Can you work these out from the model? Positions are in its coordinate system, mm. Face numbers are marked on the shaded views. A direction names the side the tool comes from. Give positions to 0.01 mm unless a question says otherwise; leave off trailing zeros. Order: outer loops, then holes, each group sorted by start corner. A loop starts at its lowest first (then second) coordinate and runs counter-clockwise, first axis right, second up.
Item 1: I want a section at A-A, the plane y = 141. Write out the boundary of the cut face in (x, z).
Item 2: If we mould it in two halves opening along X, with no side actions, what happens to the marked faces 4, 5 and 6? For each: +X half, -X half, draft (parallel to the pull), parting line (faces both ways), or undercut.
Item 3: Which directions (+Z, -Z, +X, -X, +Y, -Y) give clear straight access to the entire face, cutting with the end or side of a thin tool? Please do the marked faces 1, 2 and 3.
Item 4: If I drill on line 1 along X through (y, z) = (8, 0) (3 decimals); line 2 along Z through (x, y) = (63, 3); line 3 along Y through (x, z) = (-117, 68), over which ranges is the centre line in solid material (lowest first)?
Item 5: I'm going to push flat-ended pins straight in: pin 1 Ø10 at (y, z) = (93.5, -39.5) entering from +X; pin 2 Ø8 at (y, z) = (82.5, 90.5) entering from -X; pin 3 Ø5 at (x, z) = (109.99, 63.5) entering from +Y; pin 4 Ø6 at (y, z) = (215.5, -49) entering from +X. Where does each tip first touch, or does it pass through?
Item 6: I want a section at B-B, the plane y = 52. Write out the boundary of the cut face in (x, z), then the cut area to 3 significant figures.
```python
from build123d import *

# Parameters (mm, degrees)
SKETCH2_R           = 101.6
SKETCH2_R_2         = 69.85
SKETCH2_R_3         = 3.175
BOSS_EXTRUDE1_DEPTH = 12.7
SKETCH3_R           = 139.7
SKETCH3_R_2         = 107.95
SKETCH3_R_3         = 3.175
BOSS_EXTRUDE2_DEPTH = 12.7


with BuildPart() as part:
    # Sketch1 → Revolve1 (revolve)
    with BuildSketch(Plane.XY):
        Polygon((69.85, 279.4), (107.95, 0), (114.3, 0), (76.2, 279.4), align=None)
    revolve(axis=Axis((0, 279.4, 0), (0, -1, 0)))

    # Sketch2 → Boss-Extrude1 (add)
    with BuildSketch(Plane(origin=(0, 279.4, 0), x_dir=(1, 0, 0), z_dir=(0, 1, 0))):
        Circle(SKETCH2_R)
        Circle(SKETCH2_R_2, mode=Mode.SUBTRACT)
        with Locations((0, 88.9)):
            Circle(SKETCH2_R_3, mode=Mode.SUBTRACT)
        with Locations((44.45, 76.989658396)):
            Circle(SKETCH2_R_3, mode=Mode.SUBTRACT)
        with Locations((76.989658396, 44.45)):
            Circle(SKETCH2_R_3, mode=Mode.SUBTRACT)
        with Locations((88.9, 0)):
            Circle(SKETCH2_R_3, mode=Mode.SUBTRACT)
        with Locations((76.989658396, -44.45)):
            Circle(SKETCH2_R_3, mode=Mode.SUBTRACT)
        with Locations((44.45, -76.989658396)):
            Circle(SKETCH2_R_3, mode=Mode.SUBTRACT)
        with Locations((0, -88.9)):
            Circle(SKETCH2_R_3, mode=Mode.SUBTRACT)
        with Locations((-44.45, -76.989658396)):
            Circle(SKETCH2_R_3, mode=Mode.SUBTRACT)
        with Locations((-76.989658396, -44.45)):
            Circle(SKETCH2_R_3, mode=Mode.SUBTRACT)
        with Locations((-88.9, 0)):
            Circle(SKETCH2_R_3, mode=Mode.SUBTRACT)
        with Locations((-76.989658396, 44.45)):
            Circle(SKETCH2_R_3, mode=Mode.SUBTRACT)
        with Locations((-44.45, 76.989658396)):
            Circle(SKETCH2_R_3, mode=Mode.SUBTRACT)
    extrude(amount=-BOSS_EXTRUDE1_DEPTH)

    # Sketch3 → Boss-Extrude2 (add)
    with BuildSketch(Plane(origin=(0, 0, 0), x_dir=(-1, 0, 0), z_dir=(0, -1, 0))):
        Circle(SKETCH3_R)
        Circle(SKETCH3_R_2, mode=Mode.SUBTRACT)
        with Locations((0, 127)):
            Circle(SKETCH3_R_3, mode=Mode.SUBTRACT)
        with Locations((63.5, 109.985226281)):
            Circle(SKETCH3_R_3, mode=Mode.SUBTRACT)
        with Locations((109.985226281, 63.5)):
            Circle(SKETCH3_R_3, mode=Mode.SUBTRACT)
        with Locations((127, 0)):
            Circle(SKETCH3_R_3, mode=Mode.SUBTRACT)
        with Locations((109.985226281, -63.5)):
            Circle(SKETCH3_R_3, mode=Mode.SUBTRACT)
        with Locations((63.5, -109.985226281)):
            Circle(SKETCH3_R_3, mode=Mode.SUBTRACT)
        with Locations((0, -127)):
            Circle(SKETCH3_R_3, mode=Mode.SUBTRACT)
        with Locations((-63.5, -109.985226281)):
            Circle(SKETCH3_R_3, mode=Mode.SUBTRACT)
        with Locations((-109.985226281, -63.5)):
            Circle(SKETCH3_R_3, mode=Mode.SUBTRACT)
        with Locations((-127, 0)):
            Circle(SKETCH3_R_3, mode=Mode.SUBTRACT)
        with Locations((-109.985226281, 63.5)):
            Circle(SKETCH3_R_3, mode=Mode.SUBTRACT)
        with Locations((-63.5, 109.985226281)):
            Circle(SKETCH3_R_3, mode=Mode.SUBTRACT)
    extrude(amount=-BOSS_EXTRUDE2_DEPTH)


solid = part.part
```
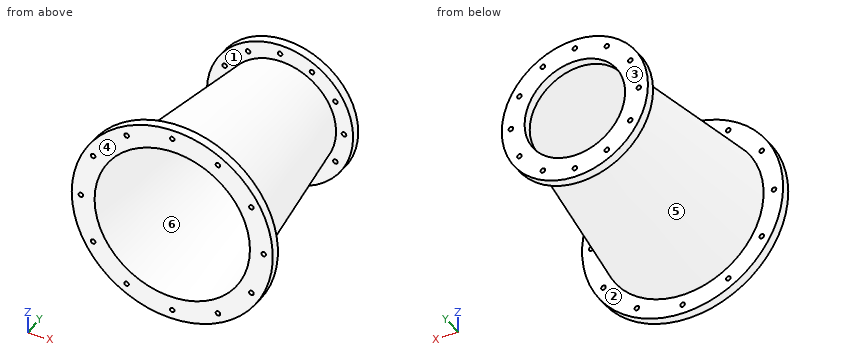
Results list:
1. outline: circle Ø190.15 at (0, 0); hole circle Ø177.45 at (0, 0)
2. face 4: draft
2. face 5: parting line
2. face 6: undercut
3. face 1: none
3. face 2: +Y
3. face 3: +Z, -Z, +X, -X, +Y
4. line 1: x = -139.7 to -130.175, -123.825 to -106.859, 106.859 to 123.825, 130.175 to 139.7
4. line 2: z = -124.69 to -113.12, -106.85 to -87.16, 87.16 to 106.85, 113.12 to 124.69
4. line 3: y = 0 to 12.7
5. pin 1: stops at x = 95.65
5. pin 2: stops at x = -56.09
5. pin 3: passes through
5. pin 4: stops at x = 71.43
6. outline: circle Ø214.42 at (0, 0); hole circle Ø201.72 at (0, 0)
6. area: 4,150 mm2
